Verification items for the finished model (mm, model axes). Face numbers are marked on the shaded views. A direction names the side the tool comes from. Give positions to 0.01 mm unless a question says otherwise; leave off trailing zeros. Order: outer loops, then holes, each group sorted by start corner. A loop starts at its lowest first (then second) coordinate and runs counter-clockwise, first axis right, second up. Notation, with made-up numbers: (27, -4) -> (57, -4) arc R4 ccw to (57, 0) -> close; hole circle Ø10 at (56.5, -30.5). An arc over 180 degrees is marked (long way). Return JSON: item names as keys, results as strings. Group by question number.
(1) Tool access check on the marked faces 5, 6 and 7. Record the directions out of +Z, -Z, +X, -X, +Y, -Y that give a thin tool (end or side, any length) a straight path to the whole face; none if there is none.
(2) Cross-section at D-D on x = -3.25. Enter the section's corners in (y, z), then the cut area to 3 significant figures.
(3) Depth check by flat-ended pin: pin 1 Ø9 at (x, z) = (-11.5, -2) entering from -Y; pin 2 Ø5 at (x, z) = (0, 0) entering from +Y; pin 3 Ø2 at (x, z) = (-11, -8.5) entering from +Y; pin 4 Ø5 at (y, z) = (11.5, 6.5) entering from -X. Enter the tip coordinate at first touch or a pass-through.
(4) Cross-section at C-C on z = -3. Enter the section's corners in (x, y), then the cut area to 3 significant figures.
(5) Release check for a two-part mould opening along Z. For the marked faces 1, 2, 3 and 4 record: pulls with the +Z half, pulls with the -Z half, needs draft (parallel to the pull), parting line crosses it, or undercut.
(6) Cross-section at B-B on y = 19.5. Enter the section's corners in (x, z), then the cut area to 3 significant figures.
(7) Thickness scan on line 1 along Z through (x, y) = (-11, 20.05); line 2 along X through (y, z) = (21.4, -8.5); line 3 along Y through (x, z) = (-8.5, 1). Record the ranges inside material, lowest first.
(8) Cross-section at A-A on x = 11. Enter the section's corners in (y, z) (3 decimals).
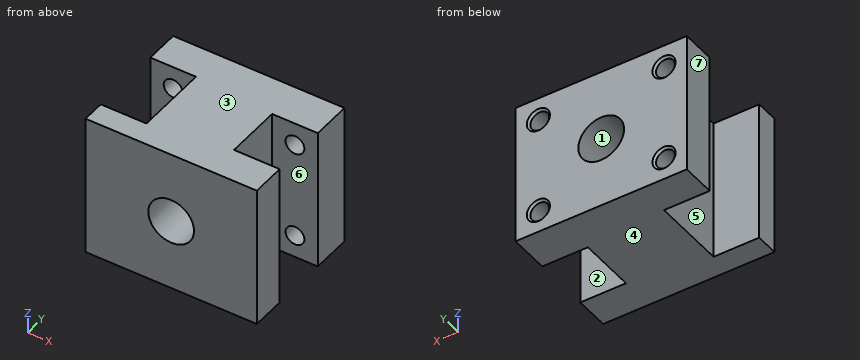
from build123d import *

# Parameters (mm, degrees)
RESSALTO_EXTRUS_O1_DEPTH = 12.5
F_8_0MM_DOWEL_HOLE1_D    = 8


# Read off the part's stored shape, not the designer's step: Furo roscado de M4x0.71
with BuildPart() as part:
    # Esboço1 → Ressalto-extrusão1 (new, symmetric)
    with BuildSketch(Plane.XY):
        Polygon((-15, 0), (15, 0), (15, 6), (7, 6), (7, 16), (15, 16), (15, 23), (-15, 23), (-15, 17), (-7, 17), (-7, 4), (-15, 4), align=None)
    extrude(amount=RESSALTO_EXTRUS_O1_DEPTH, both=True)

    # Furo roscado de M4x0.71 outline → Furo roscado de M4x0.71 (revolve, cut)
    with BuildSketch(Plane(origin=(11, 0, -8.5), x_dir=(1, 0, 0), z_dir=(0, 0, 1))):
        Polygon((0, 16), (1.65, 16), (1.65, 22.625), (2.025, 23), (0, 23), align=None)
    furo_roscado_de_m4x0_71 = revolve(axis=Axis((11, 0, -8.5), (0, 1, 0)), mode=Mode.SUBTRACT)

    # Furo roscado de M4x0.71 2 outline → Furo roscado de M4x0.71 2 (revolve, cut)
    with BuildSketch(Plane(origin=(-11, 0, -8.5), x_dir=(1, 0, 0), z_dir=(0, 0, 1))):
        Polygon((0, 17), (1.65, 17), (1.65, 22.625), (2.025, 23), (0, 23), align=None)
    furo_roscado_de_m4x0_71_2 = revolve(axis=Axis((-11, 0, -8.5), (0, 1, 0)), mode=Mode.SUBTRACT)

    # Espelhar1: Furo roscado de M4x0.71, Furo roscado de M4x0.71 2 across plane
    add(furo_roscado_de_m4x0_71.mirror(Plane.XY), mode=Mode.SUBTRACT)
    add(furo_roscado_de_m4x0_71_2.mirror(Plane.XY), mode=Mode.SUBTRACT)

    # Ø8.0mm Dowel Hole1 (through all)
    with Locations(Plane(origin=(0, 23, 0), x_dir=(1, 0, 0), z_dir=(0, 1, 0))):
        with Locations((0, 0)):
            Hole(F_8_0MM_DOWEL_HOLE1_D / 2)


solid = part.part
Verdict:
{
 "1": {"face 5": "+Z, -Z, -X", "face 6": "+Z, -Z, +X", "face 7": "+Z, -Z, -X, +Y, -Y"},
 "2": {"outline": "(0, -12.5) -> (23, -12.5) -> (23, -2.33) -> (0, -2.33) -> close; (0, 2.33) -> (23, 2.33) -> (23, 12.5) -> (0, 12.5) -> close", "area": "468 mm²"},
 "3": {"pin 1": "y = 0", "pin 2": "through", "pin 3": "y = 4", "pin 4": "x = -7"},
 "4": {"outline": "(-15, 0) -> (-2.65, 0) -> (-2.65, 23) -> (-15, 23) -> (-15, 17) -> (-7, 17) -> (-7, 4) -> (-15, 4) -> close; (2.65, 0) -> (15, 0) -> (15, 6) -> (7, 6) -> (7, 16) -> (15, 16) -> (15, 23) -> (2.65, 23) -> close", "area": "384 mm²"},
 "5": {"face 1": "undercut", "face 2": "needs draft", "face 3": "pulls with the +Z half", "face 4": "pulls with the -Z half"},
 "6": {"outline": "(-15, -12.5) -> (15, -12.5) -> (15, 12.5) -> (-15, 12.5) -> close; hole circle Ø3.3 at (-11, -8.5); hole circle Ø3.3 at (-11, 8.5); hole circle Ø8 at (0, 0); hole circle Ø3.3 at (11, -8.5); hole circle Ø3.3 at (11, 8.5)", "area": "666 mm²"},
 "7": {"line 1": "-12.5 to -10.15, -6.85 to 6.85, 10.15 to 12.5", "line 2": "-15 to -12.65, -9.35 to 9.35, 12.65 to 15", "line 3": "0 to 4, 17 to 23"},
 "8": {"outline": "(0, -12.5) -> (6, -12.5) -> (6, 12.5) -> (0, 12.5) -> close; (16, -12.5) -> (23, -12.5) -> (23, -10.525) -> (22.625, -10.15) -> (16, -10.15) -> close; (16, -6.85) -> (22.625, -6.85) -> (23, -6.475) -> (23, 6.475) -> (22.625, 6.85) -> (16, 6.85) -> close; (16, 10.15) -> (22.625, 10.15) -> (23, 10.525) -> (23, 12.5) -> (16, 12.5) -> close"}
}
